CAD build for the part. Positions are in the model's coordinates, mm. Coordinates: 2 decimals unless noted, no trailing zeros. Order: outer loops, then holes, each group sorted by start corner. A loop starts at its lowest first (then second) coordinate and runs counter-clockwise, first axis right, second up. Notation, with made-up numbers: (55.25, 55) - (83.25, 55) arc R12 cw to (83.25, 59) - close; hole circle Ø10 at (7.25, 86). An arc over 180 degrees is marked (long way). Write each question's results on one line, items separated by ' | '. Start each with the question number.
Q1. Band-saw the part on A-A, the plane z = -338. Write the cut outline in (x, y) (1 decimal).
Q2. Pin check, flat tips, straight feed: P1, Ø4.5, axis at x = 0, y = 0, coming from the +Z side; P2, Ø1, axis at x = -1, z = -417.5, coming from the +Y side; P3, Ø3, axis at y = 3, z = -315, coming from the -X side. Stop position of each tip, or through.
Q3. Wall check: probe 1 along Y at (x, z) = (0, -9.25); probe 2 along Y at (x, z) = (-1, -485); probe 3 along X at (y, z) = (-0.75, -383.5). Give the ranges that are in metal, low to high.
```python
from build123d import *

# Parameters (mm, degrees)
SKETCH1_R                  = 4.7625
BOSS_EXTRUDE1_DEPTH        = 615.95
F_10_32_TAPPED_HOLE1_D     = 4.0386
F_10_32_TAPPED_HOLE1_DEPTH = 19.05
F_10_32_TAPPED_HOLE1_TIP   = 1.213317848
F_10_32_TAPPED_HOLE4_D     = 4.0386
F_10_32_TAPPED_HOLE4_DEPTH = 19.05
F_10_32_TAPPED_HOLE4_TIP   = 1.213317848


with BuildPart() as part:
    # Sketch1 → Boss-Extrude1 (new body)
    with BuildSketch(Plane.XY):
        Circle(SKETCH1_R)
    extrude(amount=-BOSS_EXTRUDE1_DEPTH)

    # #10-32 Tapped Hole1
    with Locations(Plane(origin=(0, 0, -615.95), x_dir=(-1, 0, 0), z_dir=(0, 0, -1))):
        with Locations((0, 0)):
            Hole(F_10_32_TAPPED_HOLE1_D / 2, depth=F_10_32_TAPPED_HOLE1_DEPTH)
            with Locations((0, 0, -(F_10_32_TAPPED_HOLE1_DEPTH + F_10_32_TAPPED_HOLE1_TIP / 2))):  # 118° drill point
                Cone(0, F_10_32_TAPPED_HOLE1_D / 2, F_10_32_TAPPED_HOLE1_TIP, mode=Mode.SUBTRACT)

    # #10-32 Tapped Hole4
    with Locations(Plane.XY):
        with Locations((0, 0)):
            Hole(F_10_32_TAPPED_HOLE4_D / 2, depth=F_10_32_TAPPED_HOLE4_DEPTH)
            with Locations((0, 0, -(F_10_32_TAPPED_HOLE4_DEPTH + F_10_32_TAPPED_HOLE4_TIP / 2))):  # 118° drill point
                Cone(0, F_10_32_TAPPED_HOLE4_D / 2, F_10_32_TAPPED_HOLE4_TIP, mode=Mode.SUBTRACT)


solid = part.part
```
Results below:
1) outline: circle Ø9.5 at (0, 0)
2) P1: stops at z = 0 | P2: stops at y = 4.74 | P3: stops at x = -4.52
3) probe 1: y = -4.76 to -2.02, 2.02 to 4.76 | probe 2: y = -4.66 to 4.66 | probe 3: x = -4.7 to 4.7
